Read the model definition and answer for the solid it produces. Units are mm, in the model's axes. A direction names the side the tool comes from. Give positions to 0.01 mm unless a question says otherwise; leave off trailing zeros. Order: outer loops, then holes, each group sorted by start corner. A loop starts at its lowest first (then second) coordinate and runs counter-clockwise, first axis right, second up.
```python
from build123d import *

# Parameters (mm, degrees)
SKETCH1_W                  = 146.05
SKETCH1_H                  = 76.2
BOSS_EXTRUDE1_DEPTH        = 9.652
SKETCH3_W                  = 66.802
SKETCH3_H                  = 76.2
BOSS_EXTRUDE2_DEPTH        = 3.048
FILLET1_R                  = 12.7
F_1_4_0_5_DIAMETER_HOLE1_D = 12.7


with BuildPart() as part:
    # Sketch1 → Boss-Extrude1 (new body)
    with BuildSketch(Plane(origin=(0, 0, 0), x_dir=(1, 0, 0), z_dir=(0, 1, 0))):
        Rectangle(SKETCH1_W, SKETCH1_H)
    extrude(amount=BOSS_EXTRUDE1_DEPTH)

    # Sketch3 → Boss-Extrude2 (add)
    with BuildSketch(Plane(origin=(0, 9.652, 0), x_dir=(1, 0, 0), z_dir=(0, 1, 0))):
        Rectangle(SKETCH3_W, SKETCH3_H)
    extrude(amount=BOSS_EXTRUDE2_DEPTH)

    # Fillet1
    fillet1_edges = [part.edges().sort_by_distance(p)[0] for p in [
        (73.025, 4.826, 38.1),
        (-73.025, 4.826, 38.1),
        (-73.025, 4.826, -38.1),
        (73.025, 4.826, -38.1),
    ]]
    fillet(fillet1_edges, radius=FILLET1_R)

    # 1/4 (0.5) Diameter Hole1 (through all)
    with Locations(Plane(origin=(0, 9.652, 0), x_dir=(1, 0, 0), z_dir=(0, 1, 0))):
        with Locations((-60.325, 25.4), (-60.325, -25.4), (60.325, -25.4), (60.325, 25.4)):
            Hole(F_1_4_0_5_DIAMETER_HOLE1_D / 2)


solid = part.part
```
1) Consider L1, parallel to X at y = 7, z = -25.4 (3 decimals); L2, parallel to X at y = 2, z = 28.5; L3, parallel to Z at x = 55, y = 4.5. Determine where each line is inside the solid, lowest interval first.
Final values:
L1: x = -73.025 to -66.675, -53.975 to 53.975, 66.675 to 73.025
L2: x = -72.64 to -65.87, -54.78 to 54.78, 65.87 to 72.64
L3: z = -38.1 to -28.86, -21.94 to 21.94, 28.86 to 38.1
2) The part is cut by section B-B on z = -7. Determine the outline of the cut face in (x, y) (3 decimals), and give its area (3 significant figures).
Final values:
outline: (-73.025, 0) - (73.025, 0) - (73.025, 9.652) - (33.401, 9.652) - (33.401, 12.7) - (-33.401, 12.7) - (-33.401, 9.652) - (-73.025, 9.652) - close
area: 1,610 mm2
3) A tool of negligible diameter and unlimited length cuts with its end or side. For faces 5 (the face through (-1, 6, 38.1)), 6 (the face through (53, 9.652, -1)), 7 (the face through (-33.401, 11, 1)), from which of +Z, -Z, +X, -X, +Y, -Y can it reach the whole face along a straight path? Write none if from no direction.
Final values:
face 5: +Z, +X, -X, +Y, -Y
face 6: +Z, -Z, +X, +Y
face 7: +Z, -Z, -X, +Y
4) The part is cut by section C-C on x = 41.5. Determine the outline of the cut face in (y, z).
Final values:
outline: (0, -38.1) - (9.65, -38.1) - (9.65, 38.1) - (0, 38.1) - close
5) Given pin 1 (1.5 mm diameter, centred on y = 11.5, z = -2.5, fed in from -X); pin 2 (8 mm diameter, centred on x = 40, z = -7, fed in from -Y); pin 3 (16.5 mm diameter, centred on x = -60.325, z = 25.4, fed in from +Y), each flat-ended and moving along its own axis, determine where each tip first touches the part or whether it passes through.
Final values:
pin 1: stops at x = -33.4
pin 2: stops at y = 0
pin 3: stops at y = 9.65
6) The part is cut by section A-A on y = 6.5. Determine the outline of the cut face in (x, z) (3 decimals).
Final values:
outline: (-73.025, -25.4) arc R12.7 ccw to (-60.325, -38.1) - (60.325, -38.1) arc R12.7 ccw to (73.025, -25.4) - (73.025, 25.4) arc R12.7 ccw to (60.325, 38.1) - (-60.325, 38.1) arc R12.7 ccw to (-73.025, 25.4) - close; hole circle Ø12.7 at (-60.325, -25.4); hole circle Ø12.7 at (-60.325, 25.4); hole circle Ø12.7 at (60.325, -25.4); hole circle Ø12.7 at (60.325, 25.4)
7) For a pull along Z with two mould halves and no side action, classify faces 1 (the face through (-69.403, 4.894, 34.281)), 2 (the face through (-1, 0, -1)), 3 (the face through (-66.19, 4.76, 27.83)), 4 (the face through (-1, 6, -38.1)) as released by +Z, released by -Z, zero draft, split by the parting line, or undercut.
Final values:
face 1: released by +Z
face 2: zero draft
face 3: undercut
face 4: released by -Z
